The drawing under review shows one solid part. Ordinate dimensions are in mm from its lowest x, y, z. A direction names the side the tool comes from. Give positions to 0.01 mm unless a question says otherwise; leave off trailing zeros. Loops run counter-clockwise (first coordinate to the right, second up) from the corner with the lowest first, then second, coordinate; pieces in that order, holes last. Notation, with made-up numbers: M 54,72.25 L 97,72.25 A18 cw 97,78.25 Z; hole C 38.5,43 d6. An arc over 180 degrees is marked long. Answer as CSV lines item,"result".
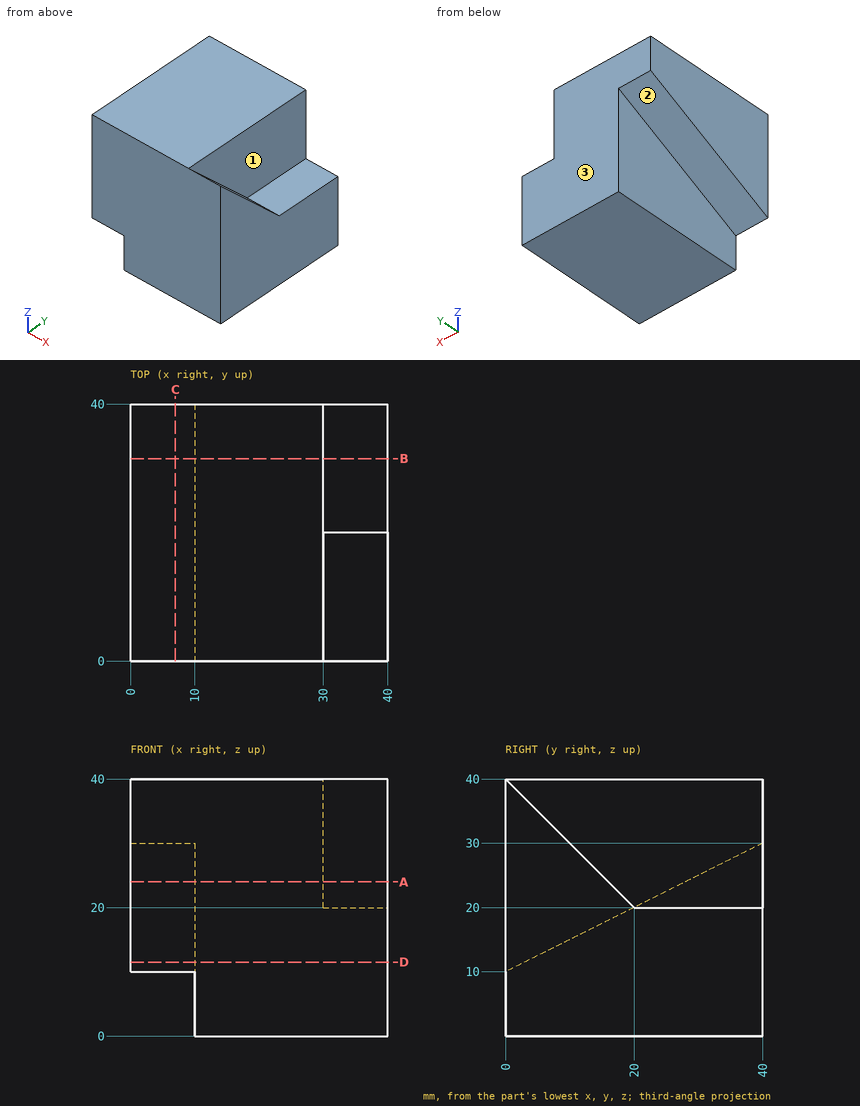
1. We need section A-A, the plane z = 24. Write out the cut boundary in (x, y).
Answer block:
outline,"M 0,0 L 40,0 L 40,16 L 30,16 L 30,40 L 10,40 L 10,28 L 0,28 Z"
2. For P1, Ø5, axis at y = 20.5, z = 30, coming from the +X side; P2, Ø1, axis at y = 18, z = 16.5, coming from the -X side; P3, Ø8, axis at x = 35, y = 26, coming from the +Z side, all flat-tipped, find the tip position at first contact; note any pin that passes through.
Answer block:
P1,"x = 30"
P2,"x = 10"
P3,"z = 20"
3. To check wall thickness, follow L1, parallel to X at y = 4, z = 10; L2, parallel to Z at x = 7.5, y = 19.5; L3, parallel to Z at x = 33.5, y = 30. State the ranges of each line that lie inside material, in increasing order. Write a range as [from, to].
Answer block:
L1,"[10, 40]"
L2,"[19.75, 40]"
L3,"[0, 20]"
4. We need section B-B, the plane y = 31.5. Write out the cut boundary in (x, z).
Answer block:
outline,"M 0,25.75 L 10,25.75 L 10,0 L 40,0 L 40,20 L 30,20 L 30,40 L 0,40 Z"
5. We need section D-D, the plane z = 11.5. Write out the cut boundary in (x, y).
Answer block:
outline,"M 0,0 L 40,0 L 40,40 L 10,40 L 10,3 L 0,3 Z"
6. We need section C-C, the plane x = 7. Write out the cut boundary in (y, z), plus the area to 3 significant figures.
Answer block:
outline,"M 0,10 L 40,30 L 40,40 L 0,40 Z"
area,"800 mm²"
7. For the marked faces 1, 2 and 3, list the 3-axis set-ups (+Z, -Z, +X, -X, +Y, -Y) from which the entire face can be reached by the end or side of a thin tool; tool diameter is ignored.
Answer block:
face 1,"+Z, +X, +Y"
face 2,"-Z, -X, +Y"
face 3,"+Z, -Z, +X, -X, +Y"
